Model file for the job. Use its own axes, mm. A direction names the side the tool comes from. Round coordinates to 2 decimals unless told otherwise and drop trailing zeros. Loops run counter-clockwise (first coordinate to the right, second up) from the corner with the lowest first, then second, coordinate; pieces in that order, holes last. Notation, with made-up numbers: (89, 42) -> (106, 42) arc R16 cw to (106, 67) -> close; hole circle Ø9 at (29.5, -24). An arc over 180 degrees is marked (long way). Use a Markdown table: item, result.
from build123d import *

# Parameters (mm, degrees)
PAD_DEPTH    = 10
POCKET_DEPTH = 4


with BuildPart() as part:
    # Sketch → Pad (new body)
    with BuildSketch(Plane.XY):
        with BuildLine():
            Line((0, 48.5), (0, 0))
            Line((0, 0), (1, 0))
            ThreePointArc((1, 0), (1.749378, 4.975062), (2, 10))
            Line((2, 10), (2, 45))
            ThreePointArc((4.5, 45), (3.25, 46.25), (2, 45))
            Line((4.5, 45), (4.5, 3))
            ThreePointArc((4.5, 3), (10.026585, -3.811222), (17.830239, 0.193634))
            ThreePointArc((17.830239, 0.193634), (17.318302, 1.511936), (16, 1))
            ThreePointArc((6.5, 3), (10.438606, -1.854122), (16, 1))
            Line((6.5, 54), (6.5, 3))
            ThreePointArc((16, 56), (10.438606, 58.854122), (6.5, 54))
            ThreePointArc((16, 56), (17.318302, 55.488064), (17.830239, 56.806366))
            ThreePointArc((17.830239, 56.806366), (10.026585, 60.811222), (4.5, 54))
            Line((4.5, 54), (4.5, 53))
            ThreePointArc((4.5, 53), (1.318019, 51.681981), (0, 48.5))
        make_face()
    extrude(amount=PAD_DEPTH)

    # Sketch001 → Pocket (cut)
    with BuildSketch(Plane(origin=(0, 0, 0), x_dir=(0, -1, 0), z_dir=(-1, 0, 0))):
        with BuildLine():
            ThreePointArc((-5.430454, 0), (-0.430454, 5), (-5.430454, 10))
            Line((-5.430454, 10), (44.569546, 10))
            Line((44.569546, 10), (44.569546, 0))
            Line((44.569546, 0), (-5.430454, 0))
        make_face()
    extrude(amount=-POCKET_DEPTH, mode=Mode.SUBTRACT)


solid = part.part
Q1. Band-saw the part on D-D, the plane z = 8. Give the cut face in (x, y).
Results list:
| item | result |
|---|---|
| outline | (0, 1.43) -> (1.27, 1.43) arc R50.5 ccw to (2, 10) -> (2, 45) arc R1.25 cw to (4.5, 45) -> (4.5, 3) arc R6.96 ccw to (17.83, 0.19) arc R1 ccw to (16, 1) arc R4.96 cw to (6.5, 3) -> (6.5, 54) arc R4.96 cw to (16, 56) arc R1 ccw to (17.83, 56.81) arc R6.96 ccw to (4.5, 54) -> (4.5, 53) arc R4.5 ccw to (0, 48.5) -> close |
Q2. Band-saw the part on C-C, the plane z = 5. Give the cut face in (x, y), plus the area to 3 significant figures.
Results list:
| item | result |
|---|---|
| outline | (0, 0.43) -> (1.09, 0.43) arc R50.5 ccw to (2, 10) -> (2, 45) arc R1.25 cw to (4.5, 45) -> (4.5, 3) arc R6.96 ccw to (17.83, 0.19) arc R1 ccw to (16, 1) arc R4.96 cw to (6.5, 3) -> (6.5, 54) arc R4.96 cw to (16, 56) arc R1 ccw to (17.83, 56.81) arc R6.96 ccw to (4.5, 54) -> (4.5, 53) arc R4.5 ccw to (0, 48.5) -> close |
| area | 286 mm² |
Q3. Pull direction Y, two halves, no side cores. Call faces 1 (the face through (1.764, 5.126, 4.93)), 2 (the face through (17.34, 1.5, 4.93)), 3 (the face through (0, 25, 5)): released by +Y, released by -Y, zero draft, split by the parting line, or undercut.
Results list:
| item | result |
|---|---|
| face 1 | released by -Y |
| face 2 | undercut |
| face 3 | zero draft |
Q4. Tool access for faces 4 (the face through (10.346, -1.834, 4.93)), 5 (the face through (6.5, 29, 5)), 6 (the face through (2, 27, 5)), 7 (the face through (0.68, 0.43, 4.89)): list every direction of +Z, -Z, +X, -X, +Y, -Y with a clear straight run to the whole face (end or side of a thin tool).
Results list:
| item | result |
|---|---|
| face 4 | +Z, -Z |
| face 5 | +Z, -Z, +X |
| face 6 | +Z, -Z, -Y |
| face 7 | -X, -Y |
Q5. Band-saw the part on B-B, the plane x = 11.75. Give the cut face in (y, z), plus the area to 3 significant figures.
Results list:
| item | result |
|---|---|
| outline | (-3.95, 0) -> (-1.95, 0) -> (-1.95, 10) -> (-3.95, 10) -> close; (58.95, 0) -> (60.95, 0) -> (60.95, 10) -> (58.95, 10) -> close |
| area | 40.0 mm² |
Q6. Drill centre lines: L1, parallel to X at y = 41, z = 2.25; L2, parallel to X at y = 1.5, z = 2.75; L3, parallel to Y at x = 13.25, z = 1.5. Where is each one in solid material? Low to high. Write a range as from..to.
Results list:
| item | result |
|---|---|
| L1 | x = 0..2, 4.5..6.5 |
| L2 | x = 0..1.28, 4.66..6.73, 16.49..17.34 |
| L3 | y = -3.73..-1.63, 58.63..60.73 |
Q7. Flat gauge pins, fed straight in: pin 1 (10 mm diameter, centred on x = 10.5, y = 33.5, fed in from +Z); pin 2 (3 mm diameter, centred on x = 2.5, z = 7.5, fed in from +Y); pin 3 (2 mm diameter, centred on x = 8.5, y = 42, fed in from -Z). Where does each tip first touch, or does it go through?
Results list:
| item | result |
|---|---|
| pin 1 | stops at z = 10 |
| pin 2 | stops at y = 52.97 |
| pin 3 | passes through |
Q8. Band-saw the part on A-A, the plane y = 30.5. Give the cut face in (x, z).
Results list:
| item | result |
|---|---|
| outline | (0, 0) -> (2, 0) -> (2, 10) -> (0, 10) -> close; (4.5, 0) -> (6.5, 0) -> (6.5, 10) -> (4.5, 10) -> close |
